Could you check a few things on this model? Use its own coordinates, in mm. Face numbers are marked on the shaded views. Coordinates: 2 decimals unless noted, no trailing zeros. Order: outer loops, then holes, each group sorted by start corner. A loop starts at its lowest first (then second) coordinate and runs counter-clockwise, first axis right, second up. Notation, with made-up numbers: (11.5, 63) - (63.5, 63) arc R20 ccw to (63.5, 85) - close; hole circle Ø5 at (2, -40). An arc over 180 degrees is marked (long way). Answer as a JSON object with one key per item and string values. Group by question number.
(1) Imagine slicing it at D-D, the plane z = 2.4. Write out the boundary of the cut face in (x, y).
(2) Please list where these lines run through material, in increasing order: probe 1 along X at (y, z) = (43.8, 1.2); probe 2 along Y at (x, z) = (-16.45, 1); probe 3 along X at (y, z) = (46, 1.3).
(3) Will these pins go through, and if not, where does the flat tip stop? P1, Ø3.5, axis at x = 17.5, y = 43, coming from the +Z side; P2, Ø0.9, axis at y = 43, z = 1, coming from the -X side; P3, Ø2.5, axis at x = -16.45, y = 43.8, coming from the +Z side; P4, Ø1.5, axis at y = 43, z = 1, coming from the +X side.
(4) Imagine slicing it at C-C, the plane y = 43.8. Write out the boundary of the cut face in (x, z).
(5) We'd pull the mould along X, two halves only. Please class the marked faces 1, 2 and 3: pulls with the +X half, pulls with the -X half, needs draft (parallel to the pull), parting line crosses it, or undercut.
(6) Imagine slicing it at B-B, the plane y = 41.75. Write out the boundary of the cut face in (x, z), and give its area (3 significant figures).
(7) Imagine slicing it at A-A, the plane x = -16.45. Write out the boundary of the cut face in (y, z).
Autodesk Inventor part; units mm, degrees
ref_plane "YZ Plane" through (0, 0, 0) normal (1, 0, 0) x (0, 1, 0)
ref_plane "XZ Plane" through (0, 0, 0) normal (0, 1, 0) x (-1, 0, 0)
ref_plane "XY Plane" through (0, 0, 0) normal (0, 0, 1) x (1, 0, 0)
sketch "Эскиз1" plane through (0, 0, 0) normal (0, 0, 1) x (1, 0, 0)
  line L0 (0, 0) -> (21.45, 0) construction
  line L1 (21.45, 0) -> (21.45, 46.7) construction
  line L2 (21.45, 46.7) -> (0, 46.7) construction
  line L3 (0, 46.7) -> (0, 0) construction
  line L4 (21.45, 46.7) -> (16.45, 46.7) construction
  line L5 (16.45, 46.7) -> (16.45, 43.8) construction
  line L6 (16.45, 43.8) -> (21.45, 43.8) construction
  line L7 (21.45, 43.8) -> (21.45, 46.7) construction
  circle A0 centre (16.45, 43.8) radius 1.5
  circle A1 centre (-16.45, 43.8) radius 1.5
  line L8 (21.45, 46.7) -> (-21.45, 46.7)
  line L9 (-21.45, 46.7) -> (-21.45, 53.5)
  line L10 (-21.45, 53.5) -> (21.45, 53.5)
  line L11 (21.45, 53.5) -> (21.45, 46.7)
  line L12 (21.45, 46.7) -> (18.95, 46.7)
  line L13 (18.95, 46.7) -> (18.95, 40.7)
  line L14 (18.95, 40.7) -> (13.95, 40.7)
  line L15 (13.95, 40.7) -> (13.95, 46.7)
  line L16 (-16.45, 46.7) -> (-16.45, 43.8) construction
  line L17 (-16.45, 43.8) -> (-21.45, 43.8) construction
  line L18 (-18.95, 46.7) -> (-18.95, 40.7)
  line L19 (-18.95, 40.7) -> (-13.95, 40.7)
  line L20 (-13.95, 40.7) -> (-13.95, 46.7)
  circle A2 centre (-16.45, 43.8) radius 1.5
  dimension "d0" = 21.45
  dimension "d1" = 46.7
  dimension "d2" = 5
  dimension "d3" = 2.9
  dimension "d4" = 3
  dimension "d5" = 42.9
  dimension "d6" = 6.8
  dimension "d7" = 2.5
  dimension "d8" = 6
  dimension "d9" = 5
extrude "Выдавливание1" add sketch "Эскиз1" along normal blind 1.5 contours L13 L14 L15 L8 | L20 L19 L18 L8
extrude "Выдавливание2" add sketch "Эскиз1" along normal blind 3 contours L8 L9 L10 L11
fillet "Сопряжение1" radius 2 4 edges at (-21.45, 50.1, 3) (-16.45, 46.7, 1.5) (21.45, 50.1, 3) (16.45, 46.7, 1.5)
properties part number "wire_fixs"
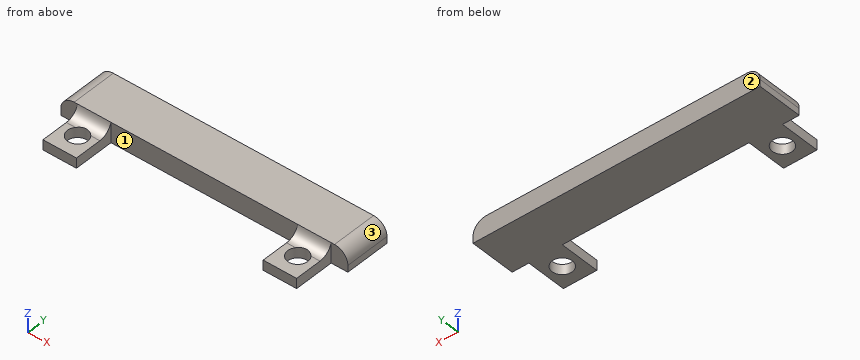
Result set:
{
 "1": {"outline": "(-20.88, 46.7) - (-18.95, 46.7) - (-18.95, 46.43) - (-13.95, 46.43) - (-13.95, 46.7) - (13.95, 46.7) - (13.95, 46.43) - (18.95, 46.43) - (18.95, 46.7) - (20.88, 46.7) - (20.88, 53.5) - (-20.88, 53.5) - close"},
 "2": {"probe 1": "x = -18.95 to -17.95, -14.95 to -13.95, 13.95 to 14.95, 17.95 to 18.95", "probe 2": "y = 40.7 to 42.3, 45.3 to 53.5", "probe 3": "x = -18.95 to -13.95, 13.95 to 18.95"},
 "3": {"P1": "stops at z = 1.5", "P2": "stops at x = -18.95", "P3": "passes through", "P4": "stops at x = 18.95"},
 "4": {"outline": "(-18.95, 0) - (-17.95, 0) - (-17.95, 1.5) - (-18.95, 1.5) - close; (-14.95, 0) - (-13.95, 0) - (-13.95, 1.5) - (-14.95, 1.5) - close; (13.95, 0) - (14.95, 0) - (14.95, 1.5) - (13.95, 1.5) - close; (17.95, 0) - (18.95, 0) - (18.95, 1.5) - (17.95, 1.5) - close"},
 "5": {"face 1": "undercut", "face 2": "needs draft", "face 3": "pulls with the +X half"},
 "6": {"outline": "(-18.95, 0) - (-13.95, 0) - (-13.95, 1.5) - (-18.95, 1.5) - close; (13.95, 0) - (18.95, 0) - (18.95, 1.5) - (13.95, 1.5) - close", "area": "15.0 mm^2"},
 "7": {"outline": "(40.7, 0) - (42.3, 0) - (42.3, 1.5) - (40.7, 1.5) - close; (45.3, 0) - (53.5, 0) - (53.5, 3) - (46.7, 3) arc R2 cw to (45.3, 1.57) - close"}
}
